Autodesk Inventor part; units mm, degrees
ref_plane "YZ Plane" through (0, 0, 0) normal (1, 0, 0) x (0, 1, 0)
ref_plane "XZ Plane" through (0, 0, 0) normal (0, 1, 0) x (-1, 0, 0)
ref_plane "XY Plane" through (0, 0, 0) normal (0, 0, 1) x (1, 0, 0)
sketch "Sketch1" plane through (0, 0, 0) normal (1, 0, 0) x (0, 1, 0)
  circle A0 centre (0, 0) radius 41
  dimension "d0" = 82
extrude "Extrusion1" add sketch "Sketch1" along normal blind 22
sketch "Sketch2" plane through (22, 0, 0) normal (1, 0, 0) x (0, 0, -1)
  circle A0 centre (0, 0) radius 11
  circle A1 centre (0, 0) radius 32
  dimension "d3" = 22
  dimension "d4" = 64
extrude "Extrusion2" cut sketch "Sketch2" against normal blind 6
sketch "Sketch3" plane through (22, 0, 0) normal (1, 0, 0) x (0, 0, -1)
  circle A0 centre (0, 0) radius 11
  dimension "d7" = 22
extrude "Extrusion3" add sketch "Sketch3" along normal blind 1.5
sketch "Sketch4" plane through (23.5, 0, 0) normal (1, 0, 0) x (0, 0, -1)
  circle A0 centre (0, 0) radius 4
  dimension "d10" = 8
extrude "Extrusion4" cut sketch "Sketch4" against normal blind 23.5
sketch "Sketch5" plane through (0, 0, 0) normal (-1, 0, 0) x (0, 0, 1)
  circle A0 centre (0, 0) radius 11
  circle A1 centre (0, 0) radius 4
  dimension "d13" = 22
  dimension "d14" = 8
extrude "Extrusion5" cut sketch "Sketch5" against normal blind 1.5
sketch "Sketch6" plane through (0, 0, 0) normal (-1, 0, 0) x (0, 0, 1)
  circle A0 centre (0, 0) radius 11
  circle A1 centre (0, 0) radius 32
  dimension "d17" = 64
  dimension "d18" = 22
extrude "Extrusion6" cut sketch "Sketch6" against normal blind 12
chamfer "Chamfer1" distance 1 angle 45 4 edges at (22, -41, 0) (0, -41, 0) (23.5, 0, 11) (1.5, 0, -11)
sketch "Sketch7" plane through (12, 0, 0) normal (-1, 0, 0) x (0, 0, 1)
  circle A0 centre (0, 0) radius 21 construction
  circle A1 centre (0, 21) radius 7
  circle A2 centre (-18.1865, 10.5) radius 7
  circle A3 centre (-18.1865, -10.5) radius 7
  circle A4 centre (0, -21) radius 7
  circle A5 centre (18.1865, -10.5) radius 7
  circle A6 centre (18.1865, 10.5) radius 7
  dimension "d24" = 42
  dimension "d25" = 14
  dimension "d28" = 360
  dimension "d30" = 10.5
extrude "Extrusion7" cut sketch "Sketch7" against normal up to next
chamfer "Chamfer2" distance 0.5 angle 45 7 edges at (16, 21, -7) (12, 21, -7) (16, 10.5, -25.1865) (12, 10.5, -25.1865) (16, -10.5, -25.1865) (12, -10.5, -25.1865) (16, 10.5, 11.1865)
chamfer "Chamfer3" distance 0.5 angle 45 4 edges at (16, -10.5, 11.1865) (12, -10.5, 11.1865) (16, -21, -7) (12, -21, -7)
fillet "Fillet1" radius 2 4 edges at (12, 0, -11) (12, 0, -32) (16, 0, 32) (16, 0, 11)
sketch "Sketch8" plane through (0, 0, 0) normal (0, 1, 0) x (-1, 0, 0)
  line L0 (0, 0) -> (-2.5, 0) construction
  line L1 (-2.5, -11) -> (-2.5, 11)
  line L2 (-2.5, 0) -> (-6.5, 0) construction
  circle A0 centre (-6.5, 0) radius 1.5
  dimension "d40" = 4
  dimension "d41" = 3
extrude "Extrusion8" cut sketch "Sketch8" along normal blind 12
thread "Thread1"
properties part number "flywheel" material "Iron, Cast"
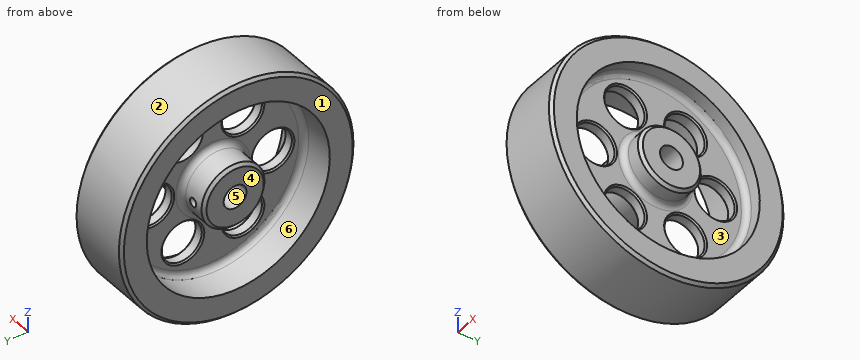
Design review of the part built by this model. Coordinates are the model's own, in mm. Face numbers are marked on the shaded views. A direction names the side the tool comes from. Coordinates: 2 decimals unless noted, no trailing zeros. Answer as a JSON object with one key per item and string values.
Q1. Take a section at A-A on y = 9. Give the number of separate pieces and of enclosed holes in the cut face, plus the area to 3 significant figures.
Answer block:
{"separate pieces": "3", "enclosed holes": "1", "area": "768 mm^2"}
Q2. Tool access review of the marked faces 5 and 6: name each direction out of +Z, -Z, +X, -X, +Y, -Y from which nothing blocks a thin tool from reaching the whole face with its end or side.
Answer block:
{"face 5": "+X, -X", "face 6": "-X"}
Q3. The part is to be moulded in two halves that separate along Y. For the marked faces 1, 2, 3 and 4, say which applies: +Y half, -Y half, draft (parallel to the pull), parting line (faces both ways), or undercut.
Answer block:
{"face 1": "draft", "face 2": "parting line", "face 3": "undercut", "face 4": "undercut"}
Q4. Clearance check with flat-ended pins moving along their axes: pin 1 Ø4 at (x, y) = (17.5, -28.5) entering from +Z (3 decimals); pin 2 Ø10 at (y, z) = (15, 11.5) entering from +X; pin 3 Ø18 at (y, z) = (21, 0) entering from +X; pin 4 Ø12.5 at (y, z) = (-10.5, -18.19) entering from -X. State where each tip first meets the part, or that it passes through.
Answer block:
{"pin 1": "stops at z = 31.285", "pin 2": "stops at x = 16", "pin 3": "stops at x = 16.27", "pin 4": "passes through"}
Q5. To check wall thickness, follow L1, parallel to X at y = 9, z = 0; L2, parallel to Y at x = 1.75, z = -9; L3, parallel to Y at x = 18.75, z = 18. State the ranges of each line that lie inside material, in increasing order.
Answer block:
{"L1": "x = 1.5 to 5, 8 to 23.5", "L2": "y = -40 to -30.71, -4.91 to 4.91, 30.71 to 40", "L3": "y = -36.84 to -26.46, 26.46 to 36.84"}
